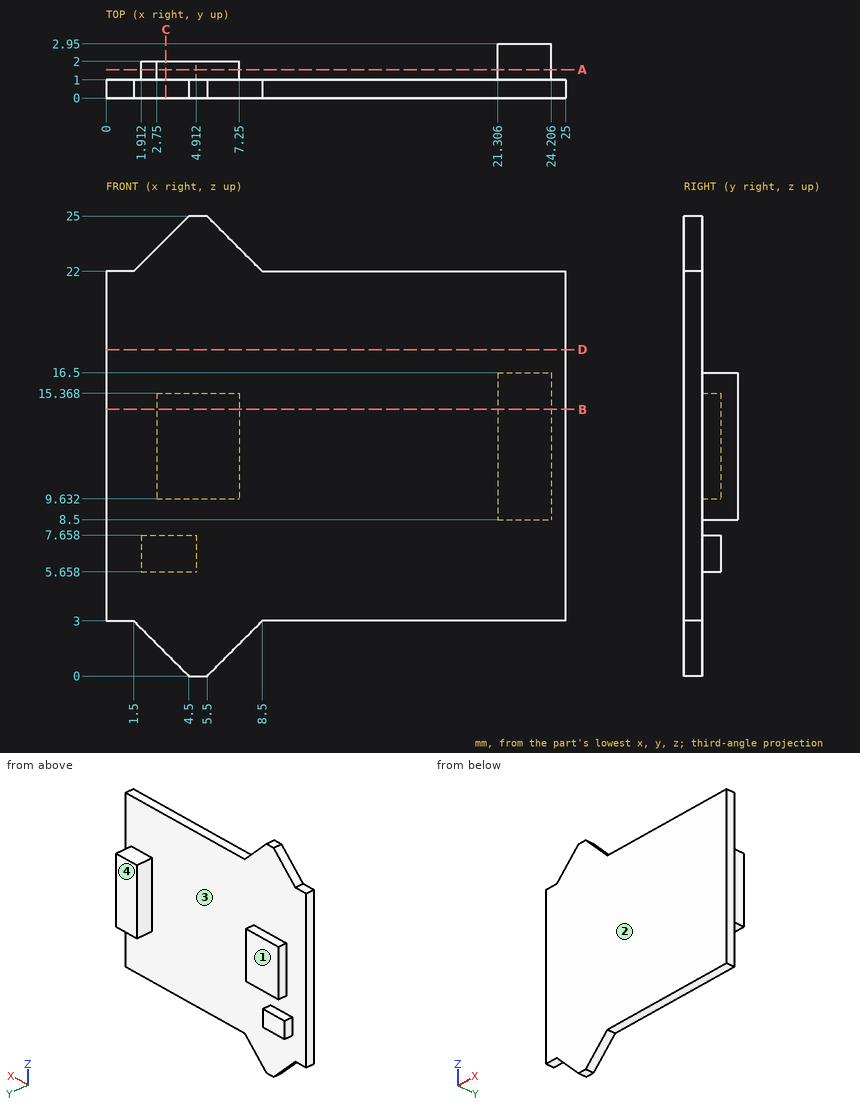
Design review of the part shown in the three views and the two pictorial views. Dimensions are in mm from the part's minimum x, y and z. A direction names the side the tool comes from. Give positions to 0.01 mm unless a question says otherwise; leave off trailing zeros. Loops run counter-clockwise (first coordinate to the right, second up) from the corner with the lowest first, then second, coordinate; pieces in that order, holes last. Notation, with made-up numbers: (22, 73.5) - (40, 73.5) arc R14 ccw to (40, 93.5) - close; hole circle Ø2 at (48.25, -22). An arc over 180 degrees is marked (long way). Answer as a JSON object with one key per item and string values.
Q1. Add section C-C on x = 3.25. State the section outline as (y, z) points.
Worked out:
{"outline": "(0, 1.25) - (1, 1.25) - (1, 5.66) - (2, 5.66) - (2, 7.66) - (1, 7.66) - (1, 9.63) - (2, 9.63) - (2, 15.37) - (1, 15.37) - (1, 23.75) - (0, 23.75) - close"}
Q2. Mouldability with a two-part tool opening along X and no side actions: class the marked faces 3 and 4 as +X half, -X half, draft (parallel to the pull), parting line (faces both ways), or undercut.
Worked out:
{"face 3": "undercut", "face 4": "draft"}
Q3. To check wall thickness, follow line 1 along Z through (x, y) = (14.5, 0.4); line 2 along Y through (x, z) = (9.5, 5); line 3 along X through (y, z) = (1.2, 5.75). State the ranges of each line that lie inside material, in increasing order.
Worked out:
{"line 1": "z = 3 to 22", "line 2": "y = 0 to 1", "line 3": "x = 1.91 to 4.91"}
Q4. Add section B-B on z = 14.5. State the section outline as (x, y) points.
Worked out:
{"outline": "(0, 0) - (25, 0) - (25, 1) - (24.21, 1) - (24.21, 2.95) - (21.31, 2.95) - (21.31, 1) - (7.25, 1) - (7.25, 2) - (2.75, 2) - (2.75, 1) - (0, 1) - close"}
Q5. Insertion check: pin 1 (0.5 mm diameter, centred on y = 1.5, z = 6.5, fed in from -X); pin 2 (0.8 mm diameter, centred on x = 17, y = 0.5, fed in from -Z); pin 3 (5 mm diameter, centred on x = 14, z = 5, fed in from -Y); pin 4 (0.8 mm diameter, centred on x = 3, y = 1.5, fed in from -Z). Each pin has a flat end and moves straight along its axis. Give the tip position at first contact, or say it passes through.
Worked out:
{"pin 1": "stops at x = 1.91", "pin 2": "stops at z = 3", "pin 3": "stops at y = 0", "pin 4": "stops at z = 5.66"}
Q6. For the marked faces 1 and 2, list the 3-axis set-ups (+Z, -Z, +X, -X, +Y, -Y) from which the entire face can be reached by the end or side of a thin tool; tool diameter is ignored.
Worked out:
{"face 1": "+Z, -Z, -X, +Y", "face 2": "+Z, -Z, +X, -X, -Y"}
Q7. Add section A-A on y = 1.55. State the section outline as (x, z) points.
Worked out:
{"outline": "(1.91, 5.66) - (4.91, 5.66) - (4.91, 7.66) - (1.91, 7.66) - close; (2.75, 9.63) - (7.25, 9.63) - (7.25, 15.37) - (2.75, 15.37) - close; (21.31, 8.5) - (24.21, 8.5) - (24.21, 16.5) - (21.31, 16.5) - close"}
Q8. Add section D-D on z = 17.75. State the section outline as (x, y) points.
Worked out:
{"outline": "(0, 0) - (25, 0) - (25, 1) - (0, 1) - close"}
